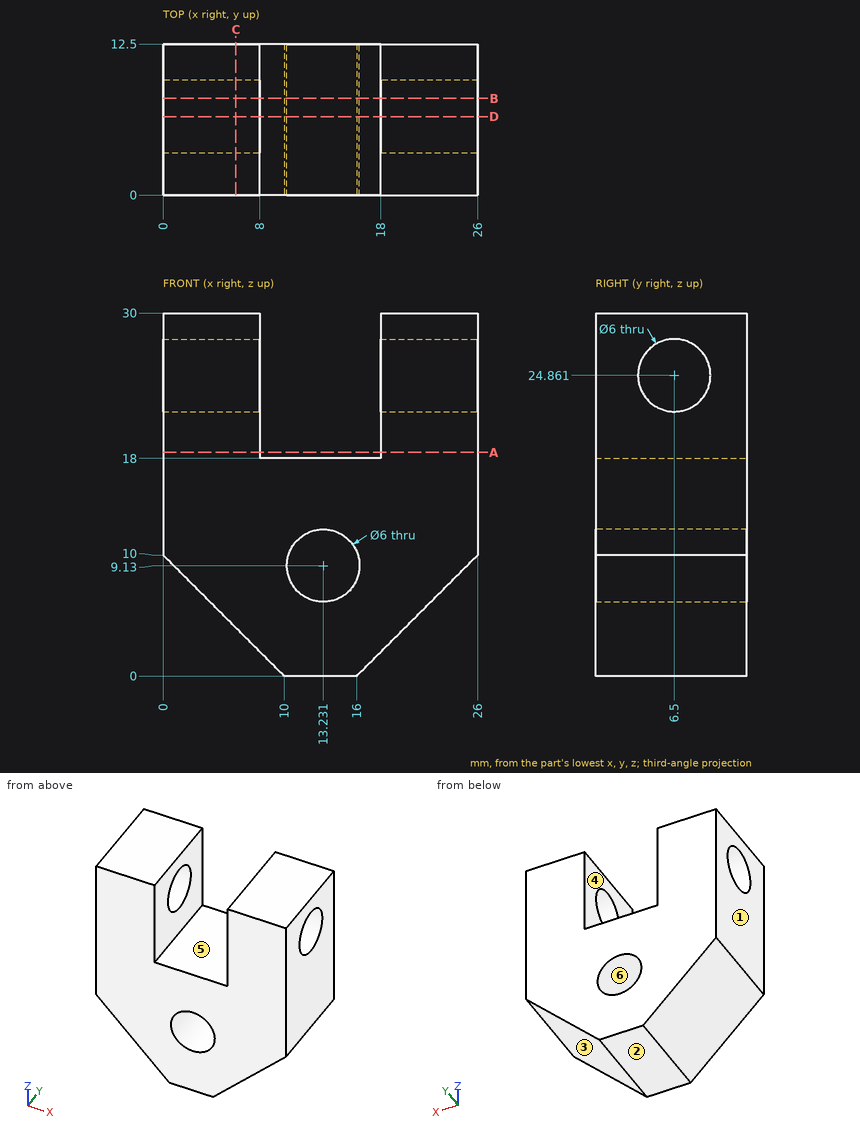
Job drawing, mm, ordinate dimensions from the low corner. One solid piece. A direction names the side the tool comes from. Give positions to 0.01 mm unless a question says otherwise; leave off trailing zeros. Write each loop counter-clockwise with the first axis right and the second up, starting at its lowest first coordinate (ties: lowest second). Pieces come first, ordered by that corner, then holes. Notation, with made-up numbers: M 37,-20 L 56,-20 A37 cw 56,17 Z; hole C 30,-22 d11. An arc over 180 degrees is marked long. Put each result on its own line as item: value. Start each with the question number.
(1) Probe L1, parallel to X at y = 3.75, z = 18.5; L2, parallel to Z at x = 2, y = 6.5; L3, parallel to Y at x = 20.5, z = 26.5. List the from-to ranges inside material, lowest first.
(2) Mould opens along X. For the marked faces 1, 2, 3 and 4 say: +X half, -X half, draft (parallel to the pull), parting line (faces both ways), or undercut.
(3) Band-saw the part on D-D, the plane y = 6.5. Write the cut outline in (x, z).
(4) Flat gauge pins, fed straight in: pin 1 Ø5.5 at (y, z) = (6.5, 24.86) entering from -X; pin 2 Ø3 at (y, z) = (4.5, 3.5) entering from +X; pin 3 Ø1 at (x, y) = (20, 3) entering from -Z. Where does each tip first touch, or does it go through?
(5) Band-saw the part on C-C, the plane x = 6. Write the cut outline in (y, z).
(6) Which spindle directions (+Z, -Z, +X, -X, +Y, -Y) get a long thin tool onto all of the face, cutting with end or side? Do the marked faces 5 and 6. Say none if no direction does.
(7) Band-saw the part on B-B, the plane y = 8. Write the cut outline in (x, z).
(8) Band-saw the part on A-A, the plane z = 18.5. Write the cut outline in (x, y), and give its area (3 significant figures).
Response values:
1. L1: x = 0 to 8, 18 to 26
1. L2: z = 8 to 21.86, 27.86 to 30
1. L3: y = 0 to 3.99, 9.01 to 12.5
2. face 1: -X half
2. face 2: draft
2. face 3: +X half
2. face 4: undercut
3. outline: M 0,10 L 10,0 L 16,0 L 26,10 L 26,21.86 L 18,21.86 L 18,18 L 8,18 L 8,21.86 L 0,21.86 Z; M 0,27.86 L 8,27.86 L 8,30 L 0,30 Z; M 18,27.86 L 26,27.86 L 26,30 L 18,30 Z; hole C 13.23,9.13 d6
4. pin 1: passes through
4. pin 2: stops at x = 21
4. pin 3: stops at z = 3.5
5. outline: M 0,4 L 12.5,4 L 12.5,30 L 0,30 Z; hole C 6.5,24.86 d6
6. face 5: +Z, +Y, -Y
6. face 6: +Y, -Y
7. outline: M 0,10 L 10,0 L 16,0 L 26,10 L 26,22.26 L 18,22.26 L 18,18 L 8,18 L 8,22.26 L 0,22.26 Z; M 0,27.46 L 8,27.46 L 8,30 L 0,30 Z; M 18,27.46 L 26,27.46 L 26,30 L 18,30 Z; hole C 13.23,9.13 d6
8. outline: M 0,0 L 8,0 L 8,12.5 L 0,12.5 Z; M 18,0 L 26,0 L 26,12.5 L 18,12.5 Z
8. area: 200 mm2
